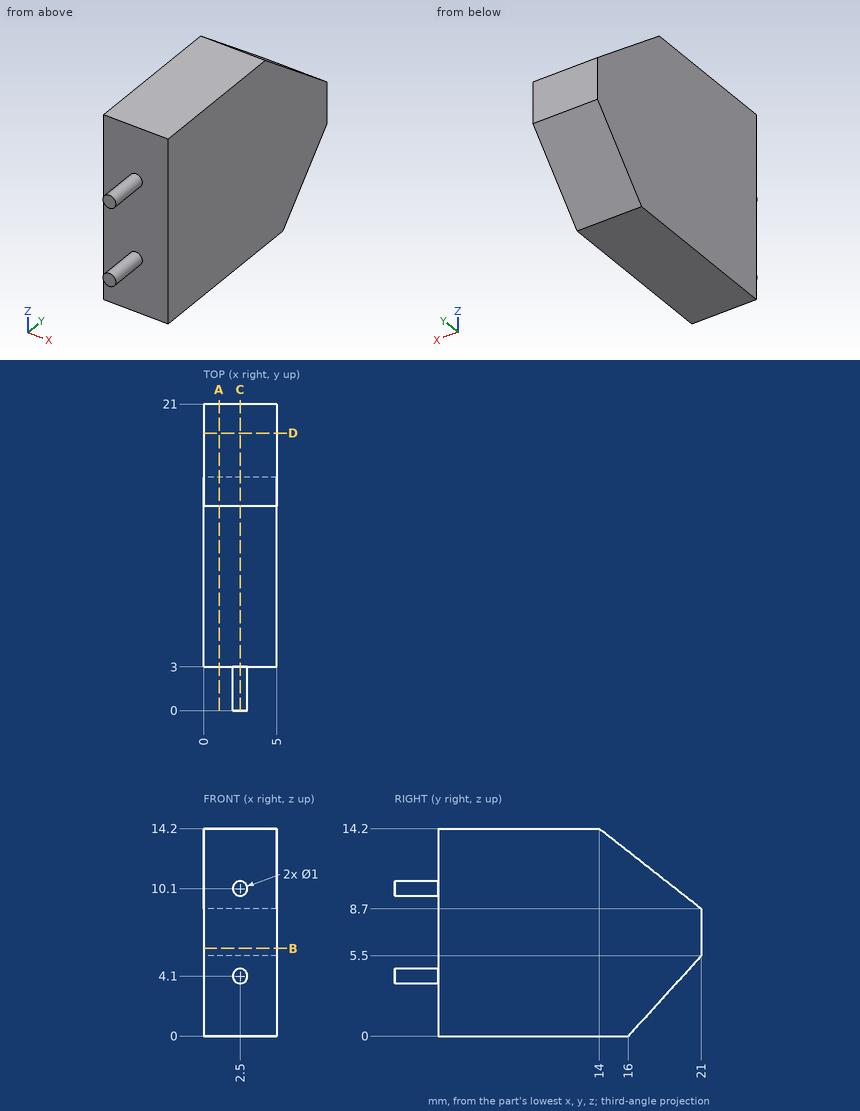
Geometry check sheet. Reference: drawing and pictorial views, mm from the part's lowest x, y, z. Give positions to 0.01 mm unless a question says otherwise; leave off trailing zeros. Loops run counter-clockwise (first coordinate to the right, second up) from the corner with the lowest first, then second, coordinate; pieces in that order, holes last. Notation, with made-up numbers: M -26,23 L -12,23 A9 cw -12,28 Z; hole C 8.25,-30 d5. An arc over 180 degrees is marked long. One line per question, with ' | ' between items.
Item 1: Section check B-B, the plane z = 6. Record the cut outline in (x, y), plus the area to 3 significant figures.
Completed:
outline: M 0,3 L 5,3 L 5,21 L 0,21 Z | area: 90.0 mm^2
Item 2: Section check D-D, the plane y = 19. Record the cut outline in (x, z).
Completed:
outline: M 0,3.3 L 5,3.3 L 5,10.27 L 0,10.27 Z
Item 3: Section check A-A, the plane x = 1.05. Record the cut outline in (y, z), plus the area to 3 significant figures.
Completed:
outline: M 3,0 L 16,0 L 21,5.5 L 21,8.7 L 14,14.2 L 3,14.2 Z | area: 223 mm^2
Item 4: Section check C-C, the plane x = 2.5. Record the cut outline in (y, z).
Completed:
outline: M 0,3.6 L 3,3.6 L 3,0 L 16,0 L 21,5.5 L 21,8.7 L 14,14.2 L 3,14.2 L 3,10.6 L 0,10.6 L 0,9.6 L 3,9.6 L 3,4.6 L 0,4.6 Z
Item 5: Thickness scan on line 1 (Y direction, x = 2.05, z = 6); line 2 (Y direction, x = 1, z = 10.5); line 3 (Z direction, x = 3.8, y = 19.75) (3 decimals). Record the ranges inside material, lowest first. Write a range as [from, to].
Completed:
line 1: y = [3, 21] | line 2: y = [3, 18.71] | line 3: z = [4.125, 9.682]
